Here's how the part is built. I have some questions about the finished solid (model axes, mm). A direction names the side the tool comes from. Coordinates: 2 decimals unless noted, no trailing zeros. Write each loop counter-clockwise with the first axis right and the second up, starting at its lowest first coordinate (ties: lowest second). Pieces come first, ordered by that corner, then holes.
(1) Imagine slicing it at D-D, the plane x = -8. List the corners of the cut face in (y, z) for me, plus the area to 3 significant figures.
(2) Imagine slicing it at C-C, the plane z = 18. List the corners of the cut face in (x, y) for me, plus the area to 3 significant figures.
(3) Thinking about a two-plate mould opening in Y: for faces 1 (the flat face through (0, 16.669, 13)), 2 (the cylindrical face through (-12.111, -15.51, 18.733)), 3 (the flat face through (10, 0, 23.114)), which applies, released by +Y, released by -Y, zero draft, split by the parting line, or undercut?
(4) Please list where these lines run through material, in increasing order: probe 1 along Y at (x, z) = (-13.5, 12); probe 2 along Z at (x, y) = (11, 9.5); probe 3 along X at (y, z) = (-8.5, 2.75).
(5) Imagine slicing it at A-A, the plane y = -7. List the corners of the cut face in (x, z) for me, plus the area to 3 significant figures.
(6) Which directions (+Z, -Z, +X, -X, +Y, -Y) give clear straight access to the entire face, cutting with the end or side of a thin tool? Please do faces 4 (the flat face through (18.433, 0, 13)), 5 (the flat face through (-16.147, 0, 3)), 6 (the flat face through (0, 0, 2.286)), 7 (the flat face through (-17, 0, 3.229)), 8 (the flat face through (0, -16.669, 13)).
(7) For pin 1 Ø6 at (y, z) = (5, 19) entering from -X; pin 2 Ø0.7 at (x, y) = (-17.5, 0) entering from +Z; pin 3 Ø1.8 at (y, z) = (4.5, 24) entering from -X, each with a flat end and sliding along its axis, tell me the tip position at first contact or that it passes through.
(8) Imagine slicing it at B-B, the plane x = 14. List the corners of the cut face in (y, z) for me.
```python
from build123d import *

# Parameters (mm, degrees)
F0_W     = 36.8659496307
F0_H     = 33.33741799
F1_DEPTH = 25.4
F2_R     = 22.1712758518
F3_T     = 2.286


# Not quite as in the source:
# - a shell that OpenCascade refuses in one call is made with other operations: the cavity is built on its own and cut out


with BuildPart() as f1:
    # F0 (on Top) → F1 (new body)
    with BuildSketch(Plane.XY):
        Rectangle(F0_W, F0_H)
    extrude(amount=F1_DEPTH)

    # F2
    f2_edges = [f1.edges().sort_by_distance(p)[0] for p in [
        (-18.432975, 0, 25.4),
    ]]
    fillet(f2_edges, radius=F2_R)

    # F3: shell of thickness 2.286, made by hand


with BuildPart() as f3_core1:
    # F3_t2: copy of F1
    add(f1.part)

    # the walls: a layer under each face that stays
    f3_faces = [f3_core1.faces().sort_by_distance(p)[0] for p in [
        (0, 16.668708995, 12.7),
        (-18.4329748154, 0, 1.6143620741),
        (0, 0, 0),
        (11.0856379259, 0, 25.4),
        (18.4329748154, 0, 12.7),
        (0, -16.668708995, 12.7),
    ]]
    thicken(f3_faces, amount=-F3_T, mode=Mode.SUBTRACT)


with BuildPart() as f1_1:
    add(f1.part)

    # what is left inside the walls is the cavity
    f3_cavity = [f3_core1.part.solids().sort_by_distance(p)[0] for p in [
        (-11.922994, 4.794236, 18.890019),
    ]]
    add(f3_cavity, mode=Mode.SUBTRACT)


solid = f1_1.part
```
Recorded:
1. outline: (-16.67, 0) - (16.67, 0) - (16.67, 22.04) - (14.38, 22.04) - (14.38, 2.29) - (-14.38, 2.29) - (-14.38, 22.04) - (-16.67, 22.04) - close
1. area: 167 mm2
2. outline: (-12.8, -16.67) - (18.43, -16.67) - (18.43, 16.67) - (-12.8, 16.67) - (-12.8, 14.38) - (16.15, 14.38) - (16.15, -14.38) - (-12.8, -14.38) - close
2. area: 209 mm2
3. face 1: released by +Y
3. face 2: zero draft
3. face 3: undercut
4. probe 1: y = -16.67 to -14.38, 14.38 to 16.67
4. probe 2: z = 0 to 2.29, 23.11 to 25.4
4. probe 3: x = -18.43 to -16.15, 16.15 to 18.43
5. outline: (-18.43, 0) - (18.43, 0) - (18.43, 25.4) - (3.74, 25.4) - (3.74, 23.11) - (16.15, 23.11) - (16.15, 2.29) - (-16.15, 2.29) - (-16.15, 3.23) - (-18.43, 3.23) - close
5. area: 168 mm2
6. face 4: +Z, -Z, +X, +Y, -Y
6. face 5: +Z
6. face 6: none
6. face 7: +Z, -X
6. face 8: +Z, -Z, +X, -X, -Y
7. pin 1: stops at x = 16.15
7. pin 2: stops at z = 3.23
7. pin 3: stops at x = 3.74
8. outline: (-16.67, 0) - (16.67, 0) - (16.67, 25.4) - (-16.67, 25.4) - close; hole (-14.38, 2.29) - (14.38, 2.29) - (14.38, 23.11) - (-14.38, 23.11) - close
